Build history of the part. All positions in model axes, mm. Face numbers are marked on the shaded views. Round coordinates to 2 decimals unless told otherwise and drop trailing zeros. Write each loop counter-clockwise with the first axis right and the second up, starting at its lowest first coordinate (ties: lowest second). Pieces come first, ordered by that corner, then holes. Notation, with made-up numbers: (57.5, 1) -> (108.5, 1) arc R31 ccw to (108.5, 35) -> close; hole circle Ø7 at (10, 39). An arc over 180 degrees is marked (long way). One line per question, with ' | ' between items.
from build123d import *

# Parameters (mm, degrees)
SKETCH1_W                   = 20
SKETCH1_H                   = 40
BOSS_EXTRUDE1_DEPTH         = 7.5
FILLET1_R                   = 5
M5_TAPPED_HOLE1_D           = 4.2
M5_TAPPED_HOLE1_CSINK_D     = 5.05
M5_TAPPED_HOLE1_CSINK_ANGLE = 90
M8_TAPPED_HOLE1_D           = 6.8
M8_TAPPED_HOLE1_DEPTH       = 20
M8_TAPPED_HOLE1_CSINK_D     = 8.05
M8_TAPPED_HOLE1_CSINK_ANGLE = 90
M8_TAPPED_HOLE1_TIP         = 2.042926105


with BuildPart() as part:
    # Sketch1 → Boss-Extrude1 (new, symmetric)
    with BuildSketch(Plane.XY):
        Rectangle(SKETCH1_W, SKETCH1_H)
    extrude(amount=BOSS_EXTRUDE1_DEPTH, both=True)

    # Fillet1
    fillet1_edges = [part.edges().sort_by_distance(p)[0] for p in [
        (10, -20, 0),
        (-10, -20, 0),
        (-10, 20, 0),
        (10, 20, 0),
    ]]
    fillet(fillet1_edges, radius=FILLET1_R)

    # M5 Tapped Hole1 (through all)
    with Locations(Plane.XY.offset(7.5)):
        with Locations((0, 12.5), (0, -12.5)):
            CounterSinkHole(M5_TAPPED_HOLE1_D / 2, M5_TAPPED_HOLE1_CSINK_D / 2, counter_sink_angle=M5_TAPPED_HOLE1_CSINK_ANGLE)

    # M8 Tapped Hole1
    with Locations(Plane.ZY.offset(10)):
        with Locations((0, 0)):
            CounterSinkHole(M8_TAPPED_HOLE1_D / 2, M8_TAPPED_HOLE1_CSINK_D / 2, depth=M8_TAPPED_HOLE1_DEPTH, counter_sink_angle=M8_TAPPED_HOLE1_CSINK_ANGLE)
            with Locations((0, 0, -(M8_TAPPED_HOLE1_DEPTH + M8_TAPPED_HOLE1_TIP / 2))):  # 118° drill point
                Cone(0, M8_TAPPED_HOLE1_D / 2, M8_TAPPED_HOLE1_TIP, mode=Mode.SUBTRACT)


solid = part.part
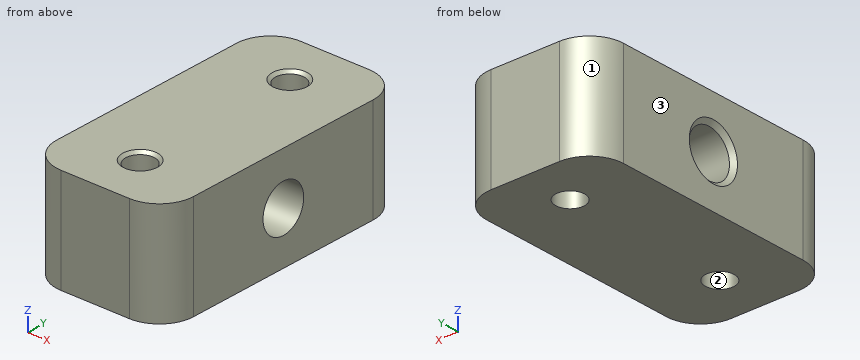
(1) Mould opens along Y. For the marked faces 1, 2 and 3 say: pulls with the +Y half, pulls with the -Y half, needs draft (parallel to the pull), parting line crosses it, or undercut.
Calculated:
face 1: pulls with the +Y half | face 2: undercut | face 3: needs draft
(2) Slice it at A-A (x = 0). Write the cut outline in (y, z) (3 decimals), then the cut area to 3 significant figures.
Calculated:
outline: (-20, -7.5) -> (-14.6, -7.5) -> (-14.6, 7.075) -> (-15.025, 7.5) -> (-20, 7.5) -> close; (-10.4, -7.5) -> (10.4, -7.5) -> (10.4, 7.075) -> (9.975, 7.5) -> (-9.975, 7.5) -> (-10.4, 7.075) -> close; (14.6, -7.5) -> (20, -7.5) -> (20, 7.5) -> (15.025, 7.5) -> (14.6, 7.075) -> close; hole circle Ø6.8 at (0, 0) | area: 437 mm2
(3) Slice it at D-D (z = -5.5). Write the cut outline in (x, y), then the cut area to 3 significant figures.
Calculated:
outline: (-10, -15) arc R5 ccw to (-5, -20) -> (5, -20) arc R5 ccw to (10, -15) -> (10, 15) arc R5 ccw to (5, 20) -> (-5, 20) arc R5 ccw to (-10, 15) -> close; hole circle Ø4.2 at (0, -12.5); hole circle Ø4.2 at (0, 12.5) | area: 751 mm2
(4) Slice it at C-C (z = 0). Write the cut outline in (x, y) (3 decimals).
Calculated:
outline: (-10, -15) arc R5 ccw to (-5, -20) -> (5, -20) arc R5 ccw to (10, -15) -> (10, -3.4) -> (-9.375, -3.4) -> (-10, -4.025) -> close; (-10, 4.025) -> (-9.375, 3.4) -> (10, 3.4) -> (10, 15) arc R5 ccw to (5, 20) -> (-5, 20) arc R5 ccw to (-10, 15) -> close; hole circle Ø4.2 at (0, -12.5); hole circle Ø4.2 at (0, 12.5)
(5) Wall check: line 1 (Y direction, x = 0, z = 5.25); line 2 (Z direction, x = -2, y = 0); line 3 (X direction, y = -12.5, z = 3). Give the ranges that are in metal, low to high. Write a range as from..to.
Calculated:
line 1: -20..-14.6, -10.4..10.4, 14.6..20 | line 2: -7.5..-3.4, 3.4..7.5 | line 3: -10..-2.1, 2.1..10
(6) Drop flat-ended pins along their axis: pin 1 (1 mm diameter, centred on x = -7, z = -0.5, fed in from +Y); pin 2 (5.5 mm diameter, centred on y = 0, z = 0, fed in from -X). Give the stop position or say it passes through.
Calculated:
pin 1: y = 19.77 | pin 2: through
(7) Slice it at B-B (y = 0). Write the cut outline in (x, z) (3 decimals), then the cut area to 3 significant figures.
Calculated:
outline: (-10, -7.5) -> (10, -7.5) -> (10, -3.4) -> (-9.375, -3.4) -> (-10, -4.025) -> close; (-10, 4.025) -> (-9.375, 3.4) -> (10, 3.4) -> (10, 7.5) -> (-10, 7.5) -> close | area: 164 mm2
